For this review, take the finished solid that the model builds, in its own axes (mm). Face numbers are marked on the shaded views. A direction names the side the tool comes from. Coordinates: 2 decimals unless noted, no trailing zeros. Order: outer loops, then holes, each group sorted by start corner. A loop starts at its lowest first (then second) coordinate and runs counter-clockwise, first axis right, second up.
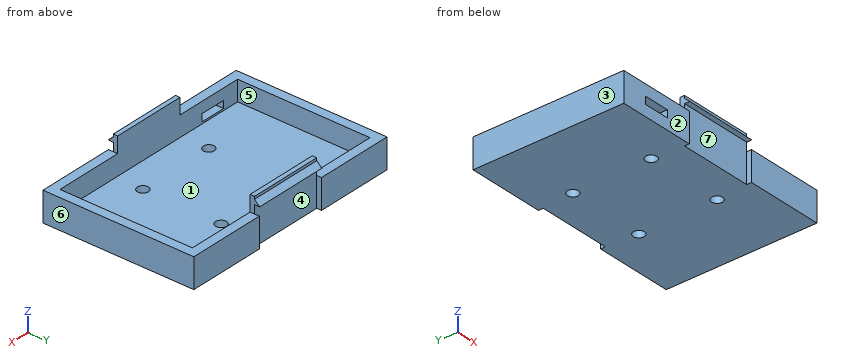
from build123d import *

# Parameters (mm, degrees)
F0_W           = 62.1
F0_H           = 40.9
F1_DEPTH       = 8
F2_T           = -2.5
F3_W           = 20
F3_H           = 12.3
F4_DEPTH       = 2.6
F5_W           = 20
F5_H           = 10.3
F6_DEPTH       = 1.4
F8_DEPTH       = 20
F9_W           = 81.3839174807
F9_H           = 28.7151690573
F10_DEPTH      = 2.501
F10_DEPTH_BACK = 9.801
F12_W          = 7
F12_H          = 2
F13_DEPTH      = 2.5
F14_R          = 1.5
F15_DEPTH      = 2.5


with BuildPart() as f1:
    # F0 (on Top) → F1 (new body)
    with BuildSketch(Plane.XY):
        Rectangle(F0_W, F0_H)
    extrude(amount=F1_DEPTH)

    # F2
    f2_openings = [f1.faces().sort_by_distance(p)[0] for p in [
        (0, 0, 8),
    ]]
    offset(amount=F2_T, openings=f2_openings)

    # F3 (on face) → F4 (join)
    with BuildSketch(Plane.XZ.offset(-17.95)):
        with Locations((0, 6.15)):
            Rectangle(F3_W, F3_H)
    extrude(amount=-F4_DEPTH)

    # F5 (on face) → F6 (cut)
    with BuildSketch(Plane(origin=(0, 20.55, 0), x_dir=(-1, 0, 0), z_dir=(0, 1, 0))):
        with Locations((0, 5.15)):
            Rectangle(F5_W, F5_H)
    extrude(amount=-F6_DEPTH, mode=Mode.SUBTRACT)

    # F7 (on face) → F8 (cut, through all)
    with BuildSketch(Plane.YZ.offset(10)):
        Polygon((19.15, 11.5828160197), (20.55, 10.3), (20.55, 12.3), (19.15, 12.3), align=None)
    extrude(amount=-F8_DEPTH, mode=Mode.SUBTRACT)

    # F9 (on face) → F10 (cut, two sides)
    with BuildSketch(Plane.XY.offset(2.5)) as f10_sk:
        with Locations((-1.038512215, -14.3575845286)):
            Rectangle(F9_W, F9_H)
    extrude(amount=-F10_DEPTH, mode=Mode.SUBTRACT)
    extrude(f10_sk.sketch, amount=F10_DEPTH_BACK, mode=Mode.SUBTRACT)

    # F11: F1 across plane


with BuildPart() as f1_1:
    add(f1.part)
    add(f1.part.mirror(Plane.XZ))

    # F12 (on face) → F13 (cut, through all)
    with BuildSketch(Plane.XZ.offset(20.45)):
        with Locations((-20.525, 4)):
            Rectangle(F12_W, F12_H)
    extrude(amount=-F13_DEPTH, mode=Mode.SUBTRACT)

    # F14 (on face) → F15 (cut, through all)
    with BuildSketch(Plane(origin=(0, 0, 0), x_dir=(1, 0, 0), z_dir=(0, 0, -1))):
        with Locations((-10.6066017178, 10.6066017178)):
            Circle(F14_R)
        with Locations((10.6066017178, 10.6066017178)):
            Circle(F14_R)
        with Locations((10.6066017178, -10.6066017178)):
            Circle(F14_R)
        with Locations((-10.6066017178, -10.6066017178)):
            Circle(F14_R)
    extrude(amount=-F15_DEPTH, mode=Mode.SUBTRACT)


solid = f1_1.part
1. Take a section at C-C, the plane x = -11. Give the boundary of the cut face in (y, z).
Answer below:
outline: (-20.45, 0) - (-12.05, 0) - (-12.05, 2.5) - (-17.95, 2.5) - (-17.95, 8) - (-20.45, 8) - close; (-9.16, 0) - (9.16, 0) - (9.16, 2.5) - (-9.16, 2.5) - close; (12.05, 0) - (20.45, 0) - (20.45, 8) - (17.95, 8) - (17.95, 2.5) - (12.05, 2.5) - close
2. Take a section at A-A, the plane x = 14. Give the boundary of the cut face in (y, z), plus the area to 3 significant figures.
Answer below:
outline: (-20.45, 0) - (20.45, 0) - (20.45, 8) - (17.95, 8) - (17.95, 2.5) - (-17.95, 2.5) - (-17.95, 8) - (-20.45, 8) - close
area: 130 mm2
3. Take a section at B-B, the plane z = 4. Give the boundary of the cut face in (x, y) (3 decimals), plus the area to 4 significant figures.
Answer below:
outline: (-31.05, -20.45) - (-24.025, -20.45) - (-24.025, -17.95) - (-28.55, -17.95) - (-28.55, 17.95) - (28.55, 17.95) - (28.55, -17.95) - (-17.025, -17.95) - (-17.025, -20.45) - (-10, -20.45) - (-10, -19.15) - (10, -19.15) - (10, -20.45) - (31.05, -20.45) - (31.05, 20.45) - (10, 20.45) - (10, 19.15) - (-10, 19.15) - (-10, 20.45) - (-31.05, 20.45) - close
area: 420.5 mm2
4. Take a section at D-D, the plane y = 14.5. Give the boundary of the cut face in (x, z).
Answer below:
outline: (-31.05, 0) - (31.05, 0) - (31.05, 8) - (28.55, 8) - (28.55, 2.5) - (-28.55, 2.5) - (-28.55, 8) - (-31.05, 8) - close
5. Machinability: for the marked faces 5, 6 and 7, which of the approach directions +Z, -Z, +X, -X, +Y, -Y give a long, thin tool a straight path to every point of the face, cutting with its end or side? Answer none if there is none.
Answer below:
face 5: +Z
face 6: +Z, -Z, +X, +Y, -Y
face 7: -Z, -Y
6. To check wall thickness, follow L1, parallel to X at y = 6, z = 3.5; L2, parallel to Y at x = 20, z = 2.75; L3, parallel to X at y = 19.5, z = 3.75. State the ranges of each line that lie inside material, in increasing order.
Answer below:
L1: x = -31.05 to -28.55, 28.55 to 31.05
L2: y = -20.45 to -17.95, 17.95 to 20.45
L3: x = -31.05 to -10, 10 to 31.05
7. The part is to be moulded in two halves that separate along Y. For the marked faces 1, 2, 3 and 4, say which applies: +Y half, -Y half, draft (parallel to the pull), parting line (faces both ways), or undercut.
Answer below:
face 1: undercut
face 2: -Y half
face 3: draft
face 4: +Y half
8. Clearance check with flat-ended pins moving along their axes: pin 1 Ø2.5 at (x, y) = (-10.61, -10.61) entering from +Z; pin 2 Ø10 at (x, y) = (-14.5, 8.5) entering from +Z; pin 3 Ø4 at (x, z) = (25, 3.5) entering from -Y; pin 4 Ø8 at (x, y) = (16.5, -16) entering from +Z. State where each tip first meets the part, or that it passes through.
Answer below:
pin 1: passes through
pin 2: stops at z = 2.5
pin 3: stops at y = -20.45
pin 4: stops at z = 8
